Can you work these out from the model? Positions are in its coordinate system, mm. Coordinates: 2 decimals unless noted, no trailing zeros. Loops run counter-clockwise (first coordinate to the right, second up) from the corner with the lowest first, then second, coordinate; pieces in that order, holes last.
Autodesk Inventor part; units mm, degrees
ref_plane "YZ Plane" through (0, 0, 0) normal (1, 0, 0) x (0, 1, 0)
ref_plane "XZ Plane" through (0, 0, 0) normal (0, 1, 0) x (-1, 0, 0)
ref_plane "XY Plane" through (0, 0, 0) normal (0, 0, 1) x (1, 0, 0)
sketch "Sketch1" plane through (0, 0, 0) normal (0, 0, 1) x (1, 0, 0)
  line L0 (0, 0) -> (0, 76.2)
  line L1 (0, 76.2) -> (25.4, 76.2)
  line L2 (25.4, 76.2) -> (76.2, 25.4)
  line L3 (76.2, 25.4) -> (76.2, 0)
  line L4 (76.2, 0) -> (0, 0)
  point P0 (12.7, 63.5)
  point P1 (12.7, 38.1)
  point P2 (12.7, 12.7)
  point P3 (38.1, 12.7)
  point P4 (63.5, 12.7)
  dimension "d0" = 76.2
  dimension "d1" = 76.2
  dimension "d2" = 25.4
  dimension "d3" = 25.4
  dimension "d4" = 12.7
  dimension "d5" = 12.7
  dimension "d6" = 25.4
  dimension "d7" = 25.4
  dimension "d8" = 25.4
  dimension "d9" = 25.4
extrude "Extrusion1" add sketch "Sketch1" against normal blind 3.175
hole "Hole1" at (12.7, 63.5, 0) at (12.7, 38.1, 0) at (12.7, 12.7, 0) at (38.1, 12.7, 0) at (63.5, 12.7, 0) direction (0, 0, -1) diameter 6.35 depth 25.4 tip angle 118
properties part number "common angle bracket"
Item 1: Suppose I cut it at A-A, the plane x = 63.5. Please give me the cut outline in (y, z) (3 decimals), plus the area to 3 significant figures.
Results are:
outline: (0, -3.175) - (9.525, -3.175) - (9.525, 0) - (0, 0) - close; (15.875, -3.175) - (38.1, -3.175) - (38.1, 0) - (15.875, 0) - close
area: 101 mm2
Item 2: Suppose I cut it at C-C, the plane x = 12.7. Please give me the cut outline in (y, z) (3 decimals), plus the area to 3 significant figures.
Results are:
outline: (0, -3.175) - (9.525, -3.175) - (9.525, 0) - (0, 0) - close; (15.875, -3.175) - (34.925, -3.175) - (34.925, 0) - (15.875, 0) - close; (41.275, -3.175) - (60.325, -3.175) - (60.325, 0) - (41.275, 0) - close; (66.675, -3.175) - (76.2, -3.175) - (76.2, 0) - (66.675, 0) - close
area: 181 mm2
Item 3: We'd pull the mould along Y, two halves only. Please class faces 1 (the face through (39, 0, -2)), 2 (the face through (35.423, 10.993, -1.61)), 3 (the face through (76.2, 13, -2)), 4 (the face through (15.5, 11.2, -1.6)): +Y half, -Y half, draft (parallel to the pull), parting line (faces both ways), or undercut.
Results are:
face 1: -Y half
face 2: undercut
face 3: draft
face 4: undercut
Item 4: I need wall thicknesses on line 1 along X through (y, z) = (12.7, -1.6) (3 decimals); line 2 along X through (y, z) = (11.5, -0.3). Which ranges of each line are inside material? Lowest first, please.
Results are:
line 1: x = 0 to 9.525, 15.875 to 34.925, 41.275 to 60.325, 66.675 to 76.2
line 2: x = 0 to 9.76, 15.64 to 35.16, 41.04 to 60.56, 66.44 to 76.2
